from build123d import *

# Parameters (mm, degrees)
CHAMFER1_SIZE = 0.508
FILLET1_R     = 0.508


with BuildPart() as part:
    # Sketch1 → Revolve1 (revolve)
    with BuildSketch(Plane(origin=(0, 0, 0), x_dir=(0, 0, -1), z_dir=(1, 0, 0))):
        Polygon((-71.766540521, 0), (-71.766540521, 1.992), (-71.258540521, 2.5), (-69.668678408, 2.5), (-69.668678408, 2.4), (-68.968678284, 2.4), (-68.968678284, 2.5), (-51.068678408, 2.5), (-51.068678408, 4.7625), (-31.157911357, 4.7625), (-31.157911357, 3.175), (-15.281908522, 3.175), (-15.281908522, 2.921), (-14.545308522, 2.921), (-14.545308522, 3.175), (22.508173379, 3.175), (22.508173379, 0), align=None)
    revolve(axis=Axis((0, 0, 0), (0, 0, 1)))

    # Chamfer1
    chamfer1_edges = [part.edges().sort_by_distance(p)[0] for p in [
        (0, -3.175, -22.508173379),
    ]]
    chamfer(chamfer1_edges, length=CHAMFER1_SIZE)

    # Fillet1
    fillet1_edges = [part.edges().sort_by_distance(p)[0] for p in [
        (0, -3.175, 31.157911357),
        (0, -2.5, 51.068678408),
    ]]
    fillet(fillet1_edges, radius=FILLET1_R)


solid = part.part
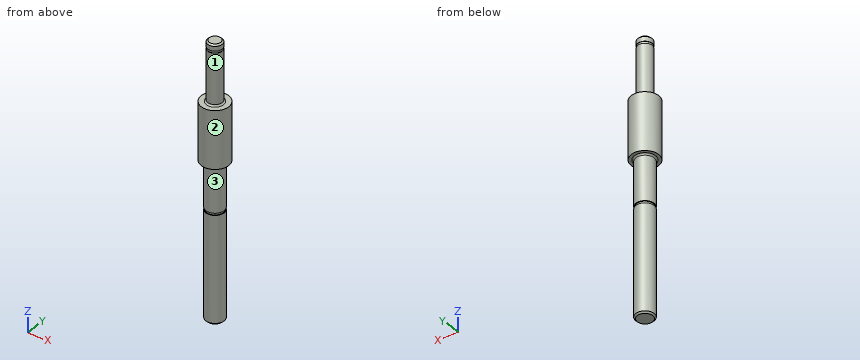
Could you check a few things on this model? Use its own coordinates, in mm. Face numbers are marked on the shaded views. A direction names the side the tool comes from. Give positions to 0.01 mm unless a question says otherwise; leave off trailing zeros. Write each loop counter-clockwise with the first axis right and the second up, starting at its lowest first coordinate (ties: lowest second). Pieces come first, ordered by that corner, then holes. Notation, with made-up numbers: (0.25, 74) - (59.25, 74) arc R19 ccw to (59.25, 80) - close; hole circle Ø5 at (7, 34.25). An arc over 180 degrees is marked (long way). Use CSV: the item, a comma, the result in double quotes. Start each with the question number.
Item 1: For the marked faces 1, 2 and 3, which set-ups out of +Z, -Z, +X, -X, +Y, -Y let a thin tool reach every point of the face, with its end or its side?
Item 2: I'm going to push flat-ended pins straight in: pin 1 (2 mm diameter, centred on x = -1.5, y = -3.5, fed in from +Z); pin 2 (4 mm diameter, centred on x = -3, y = 0.5, fed in from +Z). Where does each tip first touch, or does it pass through?
Item 3: I want a section at A-A, the plane z = 29.5. Please give me the cut outline in (x, y) (3 decimals).
Item 4: If I drill on line 1 along Z through (x, y) = (-2.75, 3.5); line 2 along X through (y, z) = (1.5, 66); line 3 along Z through (x, y) = (2.25, 2.75), over which ranges is the centre line in solid material (lowest first)?
Findings:
1,face 1,"+Z"
1,face 2,"+Z, -Z"
1,face 3,"-Z"
2,pin 1,"stops at z = 51.11"
2,pin 2,"stops at z = 71.77"
3,outline,"circle Ø6.35 at (0, 0)"
4,line 1,"z = 31.16 to 51.07"
4,line 2,"x = -2 to 2"
4,line 3,"z = 31.14 to 51.07"
